```python
from build123d import *

# Parameters (mm, degrees)
F0_W     = 381
F0_H     = 711.2
F1_DEPTH = 190.5
F2_T     = -6.35
F4_W     = 374.65
F4_H     = 698.5
F4_W_2   = 216.2134721875
F4_H_2   = 11.9601786137
F4_H_3   = 12.0113417506
F4_H_4   = 13.8943791389
F4_H_5   = 13.2367163897
F5_DEPTH = 6.35
F6_R     = 5.08
F8_DEPTH = 6.35


# Not quite as in the source:
# - a feature names something its author has since deleted; it is built from what else it names


with BuildPart() as f1:
    # F0 (on Front) → F1 (new body, symmetric)
    with BuildSketch(Plane.XZ):
        with Locations((-19.8015896951, 73.5329994828)):
            Rectangle(F0_W, F0_H)
    extrude(amount=F1_DEPTH, both=True)

    # F2
    f2_openings = [f1.faces().sort_by_distance(p)[0] for p in [
        (-19.80159, 190.5, 73.532999),
    ]]
    offset(amount=F2_T, openings=f2_openings)

    # F4 (on offset) → F5 (join, symmetric)
    with BuildSketch(Plane(origin=(0, 184.15, 0), x_dir=(-1, 0, 0), z_dir=(0, 1, 0))):
        with Locations((18.9778648138, 74.4046084881)):
            Rectangle(F4_W, F4_H)
        Polygon((-88.1409570575, 335.4734778404), (-88.1409570575, 348.0727672577), (128.07251513, 348.0727672577), (128.07251513, 335.4734778404), (128.07251513, 323.5132992268), (128.07251513, 309.8019063473), (128.07251513, 297.7905645967), (128.07251513, 286.5811288357), (128.07251513, 272.6867496967), (128.07251513, 260.7450783253), (128.07251513, 247.5083619356), (-88.1409570575, 247.5083619356), (-88.1409570575, 260.7450783253), (-88.1409570575, 272.6867496967), (-88.1409570575, 286.5811288357), (-88.1409570575, 297.7905645967), (-88.1409570575, 309.8019063473), (-88.1409570575, 323.5132992268), align=None, mode=Mode.SUBTRACT)
        with Locations((19.9657790363, 329.4933885336)):
            Rectangle(F4_W_2, F4_H_2)
        with Locations((19.9657790363, 303.796235472)):
            Rectangle(F4_W_2, F4_H_3)
        with Locations((19.9657790363, 279.6339392662)):
            Rectangle(F4_W_2, F4_H_4)
        with Locations((19.9657790363, 254.1267201304)):
            Rectangle(F4_W_2, F4_H_5)
    extrude(amount=F5_DEPTH, both=True)

    # F6
    f6_edges = [f1.edges().sort_by_distance(p)[0] for p in [
        (-19.80159, 190.5, 429.132999),
        (-19.80159, 190.5, -282.067001),
    ]]
    fillet(f6_edges, radius=F6_R)

    # F7 (on face) → F8 (cut)
    with BuildSketch(Plane(origin=(0, 190.5, 0), x_dir=(-1, 0, 0), z_dir=(0, 1, 0))):
        with BuildLine():
            ThreePointArc((-123.7823893566, 49.7743694082), (-128.773401113, 46.0705343361), (-130.1186089124, 40.0026674482))
            Line((-130.1186089124, 40.0026674482), (-108.4877372412, -114.6825799083))
            ThreePointArc((-108.4877372412, -114.6825799083), (-105.5180801987, -120.1587572974), (-99.6834033498, -122.3413996903))
            Line((-99.6834033498, -122.3413996903), (-8.89, -122.3413996903))
            ThreePointArc((-8.89, -122.3413996903), (-2.6038207153, -119.7375789751), (0, -113.4513996903))
            Line((0, -113.4513996903), (0, 73.7231935432))
            ThreePointArc((0, 73.7231935432), (-3.5472215301, 80.8286012177), (-11.3581143356, 82.2637152852))
            Line((-11.3581143356, 82.2637152852), (-123.7823893566, 49.7743694082))
        make_face()
    extrude(amount=-F8_DEPTH, mode=Mode.SUBTRACT)


solid = f1.part
```
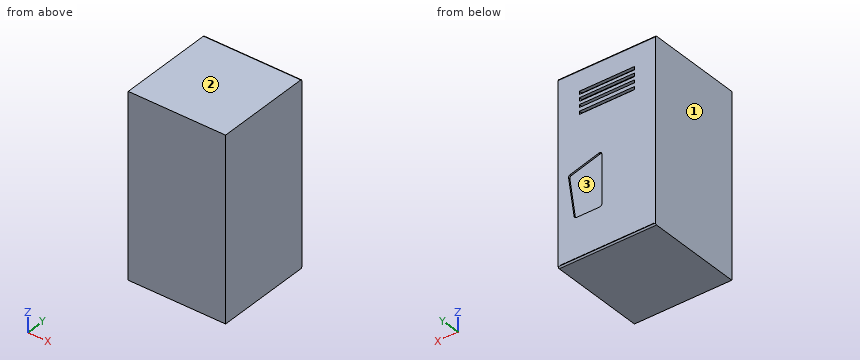
Geometry check sheet. Reference: the model listing, model coordinates, mm. Face numbers are marked on the shaded views. Round coordinates to 2 decimals unless told otherwise and drop trailing zeros. Order: outer loops, then holes, each group sorted by start corner. A loop starts at its lowest first (then second) coordinate and runs counter-clockwise, first axis right, second up. Notation, with made-up numbers: M -24.75,55 L 31.25,55 A25 cw 31.25,68 Z; hole C -21,80.25 d5. An arc over 180 degrees is marked long. Answer as CSV lines item,"result".
1) Gauge pin test, flat end, axial feed: pin 1 Ø1.5 at (x, z) = (81.5, 344) entering from +Y. Record the tip position at first contact, or that the pin passes through.
Entries:
pin 1,"y = -184.15"
2) Sectioned sample at C-C on z = 217. Record the cut outline in (x, y).
Entries:
outline,"M -210.3,-190.5 L 170.7,-190.5 L 170.7,190.5 L -210.3,190.5 Z; hole M -203.95,-184.15 L 164.35,-184.15 L 164.35,177.8 L -203.95,177.8 Z"
3) Sectioned sample at A-A on y = 6. Record the cut outline in (x, z), and give its area (3 significant figures).
Entries:
outline,"M -210.3,-282.07 L 170.7,-282.07 L 170.7,429.13 L -210.3,429.13 Z; hole M -203.95,-275.72 L 164.35,-275.72 L 164.35,422.78 L -203.95,422.78 Z"
area,"13,700 mm2"
4) Sectioned sample at B-B on x = 70. Give the number of separate pieces and of enclosed holes in the cut face, and give its area (3 significant figures).
Entries:
separate pieces,"5"
enclosed holes,"0"
area,"16,300 mm2"
5) Mould release check, pull along X, two halves, no side actions. Record for the marked faces 1, 2 and 3: +X half, -X half, draft (parallel to the pull), parting line (faces both ways), or undercut.
Entries:
face 1,"-X half"
face 2,"draft"
face 3,"undercut"
6) Sectioned sample at D-D on x = 138.5. Record the cut outline in (y, z), and give its area (3 significant figures).
Entries:
outline,"M -190.5,-282.07 L 185.42,-282.07 A5.08 ccw 190.5,-276.99 L 190.5,-275.72 L -184.15,-275.72 L -184.15,422.78 L 177.8,422.78 L 177.8,-274.85 L 190.5,-274.85 L 190.5,424.05 A5.08 ccw 185.42,429.13 L -190.5,429.13 Z"
area,"18,100 mm2"
7) Thickness scan on probe 1 along Z at (x, y) = (-95, -124); probe 2 along X at (y, z) = (-153, -199); probe 3 along Y at (x, z) = (137, -213). Record the ranges inside material, lowest first. Write a range as [from, to].
Entries:
probe 1,"[-282.07, -275.72], [422.78, 429.13]"
probe 2,"[-210.3, -203.95], [164.35, 170.7]"
probe 3,"[-190.5, -184.15], [177.8, 190.5]"
